Read the model definition and answer for the solid it produces. Units are mm, in the model's axes. A direction names the side the tool comes from. Round coordinates to 2 decimals unless told otherwise and drop trailing zeros. Order: outer loops, then holes, each group sorted by start corner. A loop starts at its lowest first (then second) coordinate and runs counter-clockwise, first axis right, second up. Notation, with made-up numbers: (59.5, 21.5) -> (90.5, 21.5) arc R10 cw to (90.5, 34.5) -> close; hole circle Ø3 at (22, 40.25). An arc over 180 degrees is marked (long way). Answer as a JSON object with one key per item and string values. Group by question number.
Item 1: Given P1, Ø8, axis at x = 3.5, z = 1, coming from the -Y side; P2, Ø1.5, axis at x = -1, z = -3, coming from the +Y side; P3, Ø3, axis at y = 6.5, z = 0, coming from the -X side, each flat-ended and moving along its own axis, determine where each tip first touches the part or whether it passes through.
Item 2: Section C-C, the plane y = 4.75 is taken. Write down the section's boundary in (x, z).
Item 3: The mould has two halves that part along X. Classify faces 4 (the flat face through (-8.486, 0.91, 2.575)), 5 (the flat face through (0, 5, 7)), 6 (the flat face through (0, 0.5, 0)): pulls with the +X half, pulls with the -X half, needs draft (parallel to the pull), parting line crosses it, or undercut.
Item 4: For faces 1 (the flat face through (-1, 5, 7.5)), 2 (the flat face through (-8.486, 0.91, -7.325)), 3 (the flat face through (-8.486, 0.899, -4.285)), determine the directions among +Z, -Z, +X, -X, +Y, -Y from which every point of the face is accessible in a straight line to the end or side of a thin tool.
Item 5: Section A-A, the plane x = 2.75 is taken. Write down the section's boundary in (y, z), plus the area to 3 significant figures.
Item 6: Consider probe 1 along X at (y, z) = (5.5, 3.5); probe 2 along Y at (x, z) = (6.75, -1). Determine where each line is inside the solid, lowest interval first. Write a range as from..to.
Item 7: Section B-B, the plane y = 3.5 is taken. Write down the section's boundary in (x, z), plus the area to 3 significant figures.
from build123d import *

# Parameters (mm, degrees)
SKETCH1_W           = 15
SKETCH1_H           = 15
BOSS_EXTRUDE1_DEPTH = 10
SHELL6_T            = -0.5
BOSS_EXTRUDE3_DEPTH = 2


with BuildPart() as part:
    # Sketch1 → Boss-Extrude1 (new body)
    with BuildSketch(Plane(origin=(0, 0, 0), x_dir=(1, 0, 0), z_dir=(0, 1, 0))):
        Rectangle(SKETCH1_W, SKETCH1_H)
    extrude(amount=BOSS_EXTRUDE1_DEPTH)

    # Shell6
    shell6_openings = [part.faces().sort_by_distance(p)[0] for p in [
        (0, 10, 0),
    ]]
    offset(amount=SHELL6_T, openings=shell6_openings, kind=Kind.INTERSECTION)

    # Sketch2 → Boss-Extrude3 (add)
    with BuildSketch(Plane.ZY.offset(7.5)):
        Polygon((-7.5, 0), (7.5, 0), (7.5, 0.5), (7.5, 10), (7, 10), (6.9, 0.5), (6.680102085, 0.5), (6.345384733, 1.309388279), (6, 0.5), (5.780102085, 0.5), (5.445384733, 1.309388279), (5.1, 0.5), (4.880102085, 0.5), (4.545384733, 1.309388279), (4.2, 0.5), (3.980102085, 0.5), (3.645384733, 1.309388279), (3.3, 0.5), (3.080102085, 0.5), (2.745384733, 1.309388279), (2.4, 0.5), (2.180102085, 0.5), (1.845384733, 1.309388279), (1.5, 0.5), (1.280102085, 0.5), (0.945384733, 1.309388279), (0.6, 0.5), (0.380102085, 0.5), (0.045384733, 1.309388279), (-0.3, 0.5), (-0.519897915, 0.5), (-0.854615267, 1.309388279), (-1.2, 0.5), (-1.419897915, 0.5), (-1.754615267, 1.309388279), (-2.1, 0.5), (-2.319897915, 0.5), (-2.654615267, 1.309388279), (-3, 0.5), (-3.219897915, 0.5), (-3.554615267, 1.309388279), (-3.9, 0.5), (-4.119897915, 0.5), (-4.454615267, 1.309388279), (-4.8, 0.5), (-5.019897915, 0.5), (-5.354615267, 1.309388279), (-5.7, 0.5), (-5.919897915, 0.5), (-6.254615267, 1.309388279), (-6.6, 0.5), (-6.819897915, 0.5), (-7.154615267, 1.309388279), (-7.5, 0.5), align=None)
    extrude(amount=BOSS_EXTRUDE3_DEPTH)


solid = part.part
Values found:
{
 "1": {"P1": "y = 0", "P2": "y = 0.5", "P3": "x = -7.5"},
 "2": {"outline": "(-9.5, 6.94) -> (-7.5, 6.94) -> (-7.5, -7.5) -> (7.5, -7.5) -> (7.5, 7.5) -> (-9.5, 7.5) -> close; hole (-7, -7) -> (7, -7) -> (7, 7) -> (-7, 7) -> close"},
 "3": {"face 4": "needs draft", "face 5": "undercut", "face 6": "undercut"},
 "4": {"face 1": "+Z, +X, -X, +Y, -Y", "face 2": "-Z, -X, +Y", "face 3": "-X, +Y"},
 "5": {"outline": "(0, -7.5) -> (10, -7.5) -> (10, -7) -> (0.5, -7) -> (0.5, 7) -> (10, 7) -> (10, 7.5) -> (0, 7.5) -> close", "area": "17.0 mm2"},
 "6": {"probe 1": "-7.5..-7, 7..7.5", "probe 2": "0..0.5"},
 "7": {"outline": "(-9.5, 6.93) -> (-7.5, 6.93) -> (-7.5, -7.5) -> (7.5, -7.5) -> (7.5, 7.5) -> (-9.5, 7.5) -> close; hole (-7, -7) -> (7, -7) -> (7, 7) -> (-7, 7) -> close", "area": "30.1 mm2"}
}
